For this review, take the finished solid that the model builds, in its own axes (mm). Face numbers are marked on the shaded views. A direction names the side the tool comes from. Round coordinates to 2 decimals unless told otherwise and drop trailing zeros. Write each loop counter-clockwise with the first axis right and the second up, starting at its lowest first coordinate (ties: lowest second). Pieces come first, ordered by that corner, then holes. Notation, with made-up numbers: M 37,62.25 L 80,62.25 A19 cw 80,66.25 Z; hole C 84,73 d10. An arc over 180 degrees is marked long. Write each question's results on one line, items separated by ' | '. Start each with the question number.
```python
from build123d import *

# Parameters (mm, degrees)
SKETCH_1_W                = 42
SKETCH_1_H                = 90
HOUSING_ENVELOPE_DEPTH    = 38
SKETCH_2_W                = 34
SKETCH_2_H                = 82
FRONT_ACCESS_WINDOW_DEPTH = 32
SKETCH_3_R                = 6.5
AXIAL_PASSAGE_DEPTH       = 107.339080304
SKETCH_4_R                = 8.3
D16_CLEARANCE_DEPTH       = 4.3


with BuildPart() as part:
    # 草图1 → Housing_envelope (new body)
    with BuildSketch(Plane.XY):
        with Locations((21, 45)):
            Rectangle(SKETCH_1_W, SKETCH_1_H)
    extrude(amount=HOUSING_ENVELOPE_DEPTH)

    # 草图2 → Front_access_window (cut)
    with BuildSketch(Plane.XY.offset(38)):
        with Locations((21, 45)):
            Rectangle(SKETCH_2_W, SKETCH_2_H)
    extrude(amount=-FRONT_ACCESS_WINDOW_DEPTH, mode=Mode.SUBTRACT)

    # 草图3 → Axial_passage (cut, through all)
    with BuildSketch(Plane(origin=(0, 90, 0), x_dir=(1, 0, 0), z_dir=(0, 1, 0))):
        with Locations(Location((21, -19, 0), (0, 0, 270))):
            Circle(SKETCH_3_R)
    extrude(amount=-AXIAL_PASSAGE_DEPTH, mode=Mode.SUBTRACT)

    # 草图4 → D16_clearance (cut)
    with BuildSketch(Plane(origin=(0, 90, 0), x_dir=(1, 0, 0), z_dir=(0, 1, 0))):
        with Locations(Location((21, -19, 0), (0, 0, 270))):
            Circle(SKETCH_4_R)
    extrude(amount=-D16_CLEARANCE_DEPTH, mode=Mode.SUBTRACT)


solid = part.part
```
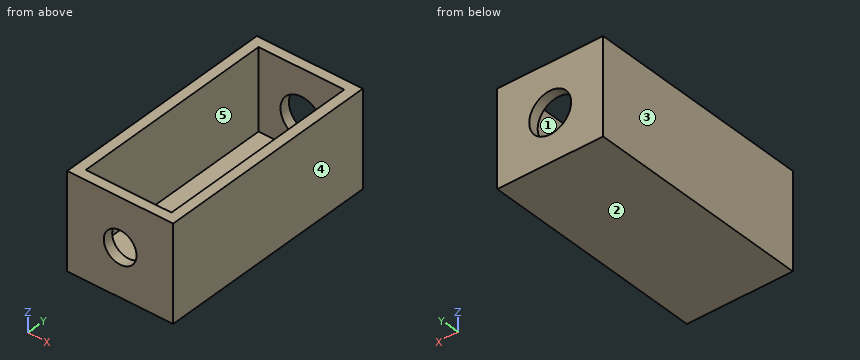
Item 1: For the marked faces 4 and 5, list the 3-axis set-ups (+Z, -Z, +X, -X, +Y, -Y) from which the entire face can be reached by the end or side of a thin tool; tool diameter is ignored.
Item 2: Insertion check: P1, Ø15, axis at x = 21, z = 19, coming from the +Y side. The pin has a flat end and moves straight along its axis. Give the tip position at first contact, or say it passes through.
Item 3: We need section D-D on z = 32.5. State the section outline as (x, y) points.
Item 4: We need section C-C on x = 21. State the section outline as (y, z) points.
Item 5: We need section A-A on z = 19. State the section outline as (x, y) points.
Item 6: For probe 1 along Y at (x, z) = (25.5, 10); probe 2 along X at (y, z) = (47, 16); probe 3 along X at (y, z) = (2.05, 19), list the stretches that pass through material, from the lowest coordinate up.
Item 7: We need section B-B on y = 83.5. State the section outline as (x, z) points, then the cut area to 3 significant figures.
Item 8: Mouldability with a two-part tool opening along X and no side actions: class the marked faces 1, 2 and 3 as pulls with the +X half, pulls with the -X half, needs draft (parallel to the pull), parting line crosses it, or undercut.
Numbers:
1) face 4: +Z, -Z, +X, +Y, -Y | face 5: +Z
2) P1: stops at y = 4
3) outline: M 0,0 L 42,0 L 42,90 L 0,90 Z; hole M 4,4 L 38,4 L 38,86 L 4,86 Z
4) outline: M 0,0 L 90,0 L 90,10.7 L 86,10.7 L 86,6 L 4,6 L 4,12.5 L 0,12.5 Z; M 0,25.5 L 4,25.5 L 4,38 L 0,38 Z; M 86,27.3 L 90,27.3 L 90,38 L 86,38 Z
5) outline: M 0,0 L 14.5,0 L 14.5,4 L 4,4 L 4,86 L 12.7,86 L 12.7,90 L 0,90 Z; M 27.5,0 L 42,0 L 42,90 L 29.3,90 L 29.3,86 L 38,86 L 38,4 L 27.5,4 Z
6) probe 1: y = 0 to 4, 86 to 90 | probe 2: x = 0 to 4, 38 to 42 | probe 3: x = 0 to 14.5, 27.5 to 42
7) outline: M 0,0 L 42,0 L 42,38 L 38,38 L 38,6 L 4,6 L 4,38 L 0,38 Z | area: 508 mm^2
8) face 1: undercut | face 2: needs draft | face 3: pulls with the -X half
